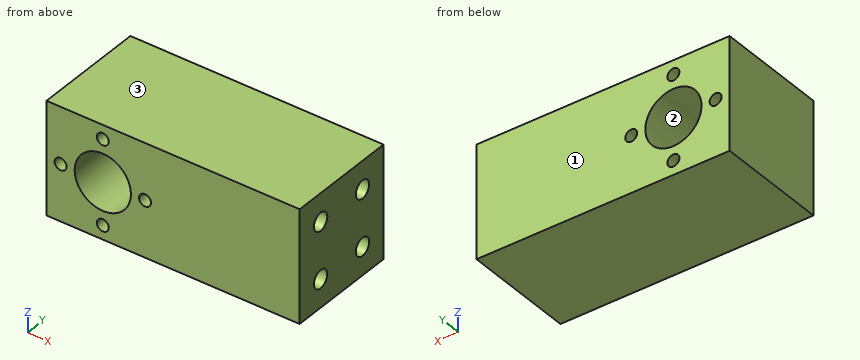
from build123d import *

# Parameters (mm, degrees)
SKETCH1_W                  = 88.9
SKETCH1_H                  = 76.2
BOSS_EXTRUDE1_DEPTH        = 12.7
SKETCH9_R                  = 6.35
CUT_EXTRUDE2_DEPTH         = 60.905780189
FILLET1_R                  = 38.1
F_10_32_TAPPED_HOLE1_D     = 4.0386
F_10_32_TAPPED_HOLE1_DEPTH = 9.652
F_10_32_TAPPED_HOLE1_TIP   = 1.213317848
CUT_EXTRUDE3_DEPTH         = 60.905780189
F_6_32_TAPPED_HOLE1_D      = 2.7051
CIRPATTERN1_COUNT          = 4


with BuildPart() as part:
    # Sketch1 → Boss-Extrude1 (new body)
    with BuildSketch(Plane(origin=(0, 0, 0), x_dir=(1, 0, 0), z_dir=(0, 1, 0))):
        Rectangle(SKETCH1_W, SKETCH1_H)
    extrude(amount=BOSS_EXTRUDE1_DEPTH)

    # Sketch9 → Cut-Extrude2 (cut, through all)
    with BuildSketch(Plane(origin=(0, 12.7, 0), x_dir=(1, 0, 0), z_dir=(0, 1, 0))):
        with Locations(Location((0, 0, 0), (0, 0, 270))):
            Circle(SKETCH9_R)
    extrude(amount=-CUT_EXTRUDE2_DEPTH, mode=Mode.SUBTRACT)

    # Fillet1
    fillet1_edges = [part.edges().sort_by_distance(p)[0] for p in [
        (-44.45, 6.35, -38.1),
        (-44.45, 6.35, 38.1),
    ]]
    fillet(fillet1_edges, radius=FILLET1_R - 0.0001)  # a hair under: the kernel refuses the full size

    # #10-32 Tapped Hole1
    with Locations(Plane(origin=(44.45, 0, 0), x_dir=(0, 0, -1), z_dir=(1, 0, 0))):
        with Locations((-6.35, 6.35), (6.35, 6.35)):
            Hole(F_10_32_TAPPED_HOLE1_D / 2, depth=F_10_32_TAPPED_HOLE1_DEPTH)
            with Locations((0, 0, -(F_10_32_TAPPED_HOLE1_DEPTH + F_10_32_TAPPED_HOLE1_TIP / 2))):  # 118° drill point
                Cone(0, F_10_32_TAPPED_HOLE1_D / 2, F_10_32_TAPPED_HOLE1_TIP, mode=Mode.SUBTRACT)

    # Sketch13 → Cut-Extrude3 (cut, through all)
    with BuildSketch(Plane(origin=(0, 12.7, 0), x_dir=(1, 0, 0), z_dir=(0, 1, 0))):
        with BuildLine():
            Line((-12.7, 12.7), (44.45, 12.7))
            Line((44.45, 12.7), (44.45, 38.1))
            Line((44.45, 38.1), (-6.35, 38.1))
            ThreePointArc((-6.35, 38.1), (-33.290768363, 26.940768363), (-44.45, 0))
            ThreePointArc((-44.45, 0), (-33.290768363, -26.940768363), (-6.35, -38.1))
            Line((-6.35, -38.1), (44.45, -38.1))
            Line((44.45, -38.1), (44.45, -12.7))
            Line((44.45, -12.7), (-12.7, -12.7))
            Line((-12.7, -12.7), (-12.7, 12.7))
        make_face()
    extrude(amount=-CUT_EXTRUDE3_DEPTH, mode=Mode.SUBTRACT)


with BuildPart() as cut_extrude3_kept_piece:
    # of the separate pieces the step leaves, the one the design keeps (cut_extrude3_pieces_kept)
    add(part.part.solids().sort_by_distance((44.45, 12.7, 12.7))[0])

    # Mirror2: Cut-Extrude3 kept piece across plane


with BuildPart() as cut_extrude3_kept_piece_1:
    add(cut_extrude3_kept_piece.part)
    add(cut_extrude3_kept_piece.part.mirror(Plane(origin=(0, 0, 0), x_dir=(0, 0, 1), z_dir=(0, -1, 0))))

    # #6-32 Tapped Hole1 (through all)
    with Locations(Plane(origin=(0, 12.7, 0), x_dir=(1, 0, 0), z_dir=(0, 1, 0))):
        with Locations((-9.525, 0)):
            f_6_32_tapped_hole1 = Hole(F_6_32_TAPPED_HOLE1_D / 2)

    # CirPattern1: #6-32 Tapped Hole1 ×4 about axis
    cirpattern1_axis = Axis((0, 0, 0), (0, 1, 0))
    for i in range(1, CIRPATTERN1_COUNT):
        add(f_6_32_tapped_hole1.rotate(cirpattern1_axis, i * 360 / CIRPATTERN1_COUNT), mode=Mode.SUBTRACT)


solid = cut_extrude3_kept_piece_1.part
Read the model definition and answer for the solid it produces. Units are mm, in the model's axes. Face numbers are marked on the shaded views. Round coordinates to 2 decimals unless told otherwise and drop trailing zeros. Write each loop counter-clockwise with the first axis right and the second up, starting at its lowest first coordinate (ties: lowest second). Pieces come first, ordered by that corner, then holes. Notation, with made-up numbers: (-11, -21) - (45, -21) arc R31 cw to (45, 8) - close; hole circle Ø6 at (12.5, -34). An arc over 180 degrees is marked (long way). One line per question, with ' | ' between items. Start each with the question number.
1. Section D-D (y = 11.25) is taken. Determine the outline of the cut face in (x, z) (3 decimals), and give its area (3 significant figures).
2. Section A-A (z = 0) is taken. Determine the outline of the cut face in (x, y), and give its area (3 significant figures).
3. This flat-tipped pin is pushed along its axis until it touches: pin 1 (3.5 mm diameter, centred on y = 6.35, z = 6.35, fed in from +X). Where does it stop, or does it pass through?
4. Section B-B (x = 0) is taken. Determine the outline of the cut face in (y, z), and give its area (3 significant figures).
5. Section C-C (x = 39) is taken. Determine the outline of the cut face in (y, z), and give its area (3 significant figures).
6. Find the intervals of material crossed by probe 1 along Z at (x, y) = (39, 6.35); probe 2 along X at (y, z) = (-7.5, 9.5), in increasing order. Write a range as [from, to].
7. For a pull along Z with two mould halves and no side action, classify the marked faces 1, 2 and 3 as +Z half, -Z half, draft (parallel to the pull), parting line (faces both ways), or undercut.
Filled in:
1) outline: (-12.7, -12.7) - (44.45, -12.7) - (44.45, 12.7) - (-12.7, 12.7) - close; hole circle Ø2.705 at (-9.525, 0); hole circle Ø12.7 at (0, 0); hole circle Ø2.705 at (0, -9.525); hole circle Ø2.705 at (0, 9.525); hole circle Ø2.705 at (9.525, 0) | area: 1,300 mm²
2) outline: (-12.7, -12.7) - (-10.88, -12.7) - (-10.88, 12.7) - (-12.7, 12.7) - close; (-8.17, -12.7) - (-6.35, -12.7) - (-6.35, 12.7) - (-8.17, 12.7) - close; (6.35, -12.7) - (8.17, -12.7) - (8.17, 12.7) - (6.35, 12.7) - close; (10.88, -12.7) - (44.45, -12.7) - (44.45, 12.7) - (10.88, 12.7) - close | area: 992 mm²
3) pin 1: x = 34.64
4) outline: (-12.7, -12.7) - (12.7, -12.7) - (12.7, -10.88) - (-12.7, -10.88) - close; (-12.7, -8.17) - (12.7, -8.17) - (12.7, -6.35) - (-12.7, -6.35) - close; (-12.7, 6.35) - (12.7, 6.35) - (12.7, 8.17) - (-12.7, 8.17) - close; (-12.7, 10.88) - (12.7, 10.88) - (12.7, 12.7) - (-12.7, 12.7) - close | area: 185 mm²
5) outline: (-12.7, -12.7) - (12.7, -12.7) - (12.7, 12.7) - (-12.7, 12.7) - close; hole circle Ø4.04 at (-6.35, -6.35); hole circle Ø4.04 at (-6.35, 6.35); hole circle Ø4.04 at (6.35, -6.35); hole circle Ø4.04 at (6.35, 6.35) | area: 594 mm²
6) probe 1: [-12.7, -8.37], [-4.33, 4.33], [8.37, 12.7] | probe 2: [-12.7, -1.35], [1.35, 44.45]
7) face 1: draft | face 2: undercut | face 3: +Z half
